from build123d import *

# Parameters (mm, degrees)
SALIENTE_EXTRUIR1_DEPTH = 2.7


with BuildPart() as part:
    # Croquis1 → Saliente-Extruir1 (new body)
    with BuildSketch(Plane.YZ):
        with BuildLine():
            Line((-55.234115884, -6.578730109), (-38.680874308, -6.578730181))
            Line((-38.680874308, -6.578730181), (-38.680874295, -3.648339402))
            Line((-38.680874295, -3.648339402), (-35.830874295, -3.648339414))
            Line((-35.830874295, -3.648339414), (-35.830874308, -6.578730194))
            Line((-35.830874308, -6.578730194), (-19.420064078, -6.578730266))
            Line((-19.420064078, -6.578730266), (-19.420064066, -3.648339486))
            Line((-19.420064066, -3.648339486), (-16.570064066, -3.648339498))
            Line((-16.570064066, -3.648339498), (-16.570064078, -6.578730278))
            Line((-16.570064078, -6.578730278), (-0.159253849, -6.57873035))
            Line((-0.159253849, -6.57873035), (-0.159253836, -3.64833957))
            Line((-0.159253836, -3.64833957), (2.690746164, -3.648339583))
            Line((2.690746164, -3.648339583), (2.690746151, -6.578730362))
            Line((2.690746151, -6.578730362), (19.101467122, -6.578730434))
            Line((19.101467122, -6.578730434), (19.101467135, -3.648339654))
            Line((19.101467135, -3.648339654), (21.951467135, -3.648339667))
            Line((21.951467135, -3.648339667), (21.951467122, -6.578730446))
            Line((21.951467122, -6.578730446), (38.36236661, -6.578730518))
            Line((38.36236661, -6.578730518), (38.362366623, -3.648339738))
            Line((38.362366623, -3.648339738), (41.212366623, -3.648339751))
            Line((41.212366623, -3.648339751), (41.21236661, -6.57873053))
            Line((41.21236661, -6.57873053), (57.62317684, -6.578730602))
            Line((57.62317684, -6.578730602), (57.623176853, -3.648339823))
            Line((57.623176853, -3.648339823), (60.473176853, -3.648339835))
            Line((60.473176853, -3.648339835), (60.47317684, -6.579394365))
            Line((60.47317684, -6.579394365), (92.691783737, -6.579394365))
            add(Edge.make_bspline(
                [(65.515708358, -0.078730637), (68.197256802, -0.258981281), (73.772414922, -0.633736737), (81.258018047, -2.465410904), (87.672687502, -4.376295676), (91.146213496, -5.900976656), (92.691783737, -6.579394365)],
                knots=[0, 0, 0, 0, 0.286390458, 0.595428587, 0.819983056, 1, 1, 1, 1], degree=3))
            Line((65.515708358, -0.078730637), (-58.084017099, -0.078730097))
            Line((-58.084017099, -0.078730097), (-58.120461042, -0.078730097))
            add(Edge.make_bspline(
                [(-66.004307996, -0.939930258), (-64.387448411, -0.680254728), (-61.772849484, -0.260337396), (-59.129262369, -0.128890612), (-58.120461042, -0.078730097)],
                knots=[0, 0, 0, 0, 0.61839679, 1, 1, 1, 1], degree=3))
            add(Edge.make_bspline(
                [(-82.084508668, -6.41226612), (-80.796356469, -5.618417967), (-78.096313761, -3.954465587), (-72.617339557, -2.219536347), (-68.499900924, -1.422817975), (-66.004307996, -0.939930258)],
                knots=[0, 0, 0, 0, 0.26437177, 0.554138766, 1, 1, 1, 1], degree=3))
            add(Edge.make_bspline(
                [(-82.308216262, -6.578730097), (-82.257659483, -6.539388838), (-82.184342615, -6.482244345), (-82.108242057, -6.428888889), (-82.084508668, -6.41226612)],
                knots=[0, 0, 0, 0, 0.688452323, 1, 1, 1, 1], degree=3))
            Line((-82.308216262, -6.578730097), (-58.084115884, -6.578730097))
            Line((-58.084115884, -6.578730097), (-58.084115884, -3.648339317))
            Line((-58.084115884, -3.648339317), (-55.234115884, -3.648339317))
            Line((-55.234115884, -3.648339317), (-55.234115884, -6.578730109))
        make_face()
    extrude(amount=SALIENTE_EXTRUIR1_DEPTH)


solid = part.part
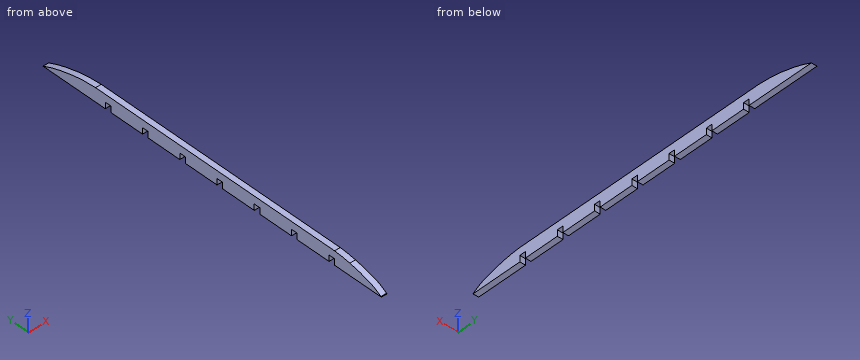
Build history of the part. All positions in model axes, mm. Coordinates: 2 decimals unless noted, no trailing zeros. Write item = value, one per line. Start each with the question number.
1) Flat gauge pins, fed straight in: pin 1 Ø1.4 at (x, z) = (1.5, -4.5) entering from +Y; pin 2 Ø0.8 at (x, z) = (2, -5) entering from +Y; pin 3 Ø1.4 at (x, z) = (2, -4.5) entering from -Y. Where does each tip first touch, or does it go through?
2) Saw through at A-A on z = -5.25. Count the separate pieces of the cut face and the enclosed holes in it, then the cut area to 3 significant figures.
3) Wall check: line 1 along Z through (x, y) = (2.1, 72.5); line 2 along Z through (x, y) = (1.1, 2.5). Give the ranges that are in metal, low to high. Write a range as from..to.
From the geometry:
q1.pin_1 = 89.47
q1.pin_2 = 89.96
q1.pin_3 = -80.07
q2.separate_pieces = 8
q2.enclosed_holes = 0
q2.area = 404 mm^2
q3.line_1 = -6.58..-0.7
q3.line_2 = -3.65..-0.08
